Verification items for this drawing (mm, ordinates from the low corner). A direction names the side the tool comes from. Give positions to 0.01 mm unless a question says otherwise; leave off trailing zeros. Write each loop counter-clockwise with the first axis right and the second up, starting at its lowest first coordinate (ties: lowest second). Pieces come first, ordered by that corner, then holes. Notation, with made-up numbers: (-39.5, 88.5) -> (-29.5, 88.5) arc R7 ccw to (-29.5, 101.5) -> close; hole circle Ø11 at (-31, 32). An arc over 180 degrees is marked (long way). Write item = value, one per line.
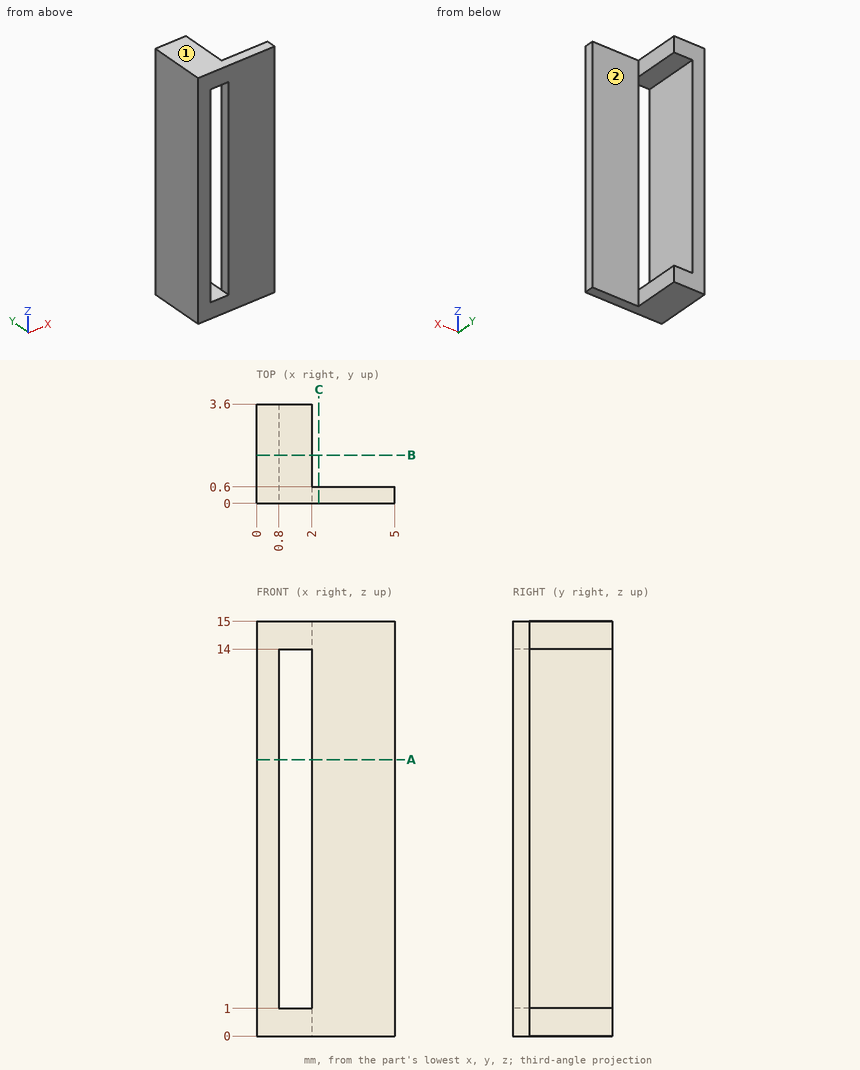
Item 1: Material ranges on line 1 (Z direction, x = 1.8, y = 2.95); line 2 (X direction, y = 0.25, z = 2.75); line 3 (Y direction, x = 3.9, z = 10), recorded low to high.
Response values:
line_1 = 0 to 1, 14 to 15
line_2 = 0 to 0.8, 2 to 5
line_3 = 0 to 0.6
Item 2: Sectioned sample at C-C on x = 2.25. Record the cut outline in (y, z).
Response values:
outline = (0, 0) -> (0.6, 0) -> (0.6, 15) -> (0, 15) -> close
Item 3: Go/stop test with flat-tipped pins: P1, Ø0.8, axis at y = 1.5, z = 14.5, coming from the +X side; P2, Ø1, axis at x = 2.5, z = 11, coming from the +Y side. Record where each tip stops, or that it passes through.
Response values:
P1 = 2
P2 = 0.6
Item 4: Sectioned sample at A-A on z = 10. Record the cut outline in (x, y).
Response values:
outline = (0, 0) -> (0.8, 0) -> (0.8, 3.6) -> (0, 3.6) -> close; (2, 0) -> (5, 0) -> (5, 0.6) -> (2, 0.6) -> close
Item 5: Sectioned sample at B-B on y = 1.75. Record the cut outline in (x, z).
Response values:
outline = (0, 0) -> (2, 0) -> (2, 1) -> (0.8, 1) -> (0.8, 14) -> (2, 14) -> (2, 15) -> (0, 15) -> close
Item 6: Set-up check for the marked faces 1 and 2: record each of +Z, -Z, +X, -X, +Y, -Y from which the full face is reachable in a straight line by a thin tool's end or side.
Response values:
face_1 = +Z, +X, -X, +Y, -Y
face_2 = +Z, -Z, +X, +Y
